Can you work these out from the model? Positions are in its coordinate system, mm. Face numbers are marked on the shaded views. A direction names the side the tool comes from. Coordinates: 2 decimals unless noted, no trailing zeros. Order: outer loops, then holes, each group sorted by start corner. A loop starts at its lowest first (then second) coordinate and runs counter-clockwise, first axis right, second up. Notation, with made-up numbers: (89, -26) -> (119, -26) arc R29 ccw to (119, 7) -> close; hole circle Ø8 at (-23, 13.5). An arc over 180 degrees is marked (long way). Answer in a Markdown table with one row per item. Add a question column.
1. Imagine slicing it at B-B on y = -21. Write out the boundary of the cut face in (x, z), plus the area to 3 significant figures.
2. Imagine slicing it at C-C on z = 4.75. Write out the boundary of the cut face in (x, y), plus the area to 3 significant figures.
3. Imagine slicing it at D-D on y = 5. Write out the boundary of the cut face in (x, z), plus the area to 3 significant figures.
4. On a 3-axis mill with a long thin cutter (end or side, diameter ignored), from which of +Z, -Z, +X, -X, +Y, -Y can I reach the whole of each face in a straight line? I mean the marked faces 1, 2, 3 and 4. Say none if no direction works.
5. Will these pins go through, and if not, where does the flat tip stop? pin 1 (6 mm diameter, centred on x = 17.5, y = -27, fed in from +Z); pin 2 (3 mm diameter, centred on x = -5.66, y = -5.66, fed in from +Z); pin 3 (1.8 mm diameter, centred on y = -2, z = 9, fed in from +X); pin 4 (3 mm diameter, centred on y = -24.5, z = 1.5, fed in from +X).
6. Imagine slicing it at A-A on x = 0. Write out the boundary of the cut face in (y, z), plus the area to 3 significant figures.
7. If I drill on line 1 along Y through (x, z) = (23.5, 22); line 2 along Z through (x, y) = (-8.5, -22); line 3 along Y through (x, z) = (-7, 4.75), over which ranges is the centre line in solid material (lowest first)? Write a range as [from, to].
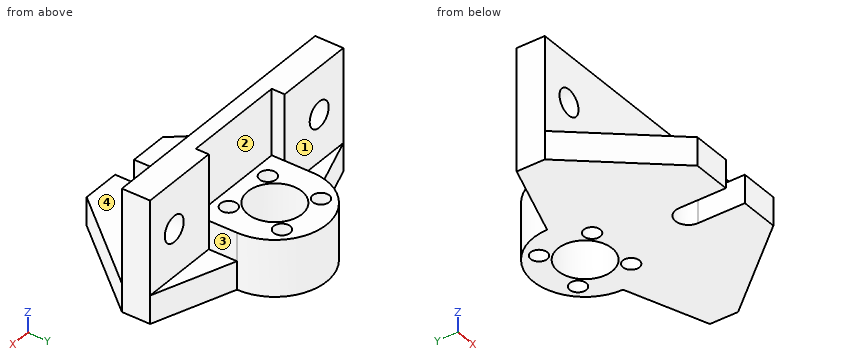
from build123d import *

# Parameters (mm, degrees)
SKETCH_R        = 5.75
SKETCH_R_2      = 1.75
PAD_DEPTH       = 26
SKETCH001_W     = 22
SKETCH001_H     = 6
PAD001_DEPTH    = 20
POCKET_DEPTH    = 6.001
PAD002_DEPTH    = 26
PAD002_FACE13_W = 20
PAD002_FACE13_H = 20
POCKET001_DEPTH = 144.217351
SKETCH004_R     = 2.75
POCKET002_DEPTH = 153.217351
POCKET003_DEPTH = 14
PAD003_DEPTH    = 6


with BuildPart() as part:
    # Sketch → Pad (new body)
    with BuildSketch(Plane.XY):
        with BuildLine():
            ThreePointArc((11, 0), (0, 11), (-11, 0))
            Line((-11, 0), (-11, -12))
            Line((11, -12), (-11, -12))
            Line((11, -12), (11, 0))
        make_face()
        Circle(SKETCH_R, mode=Mode.SUBTRACT)
        with Locations((-5.656854, 5.656854)):
            Circle(SKETCH_R_2, mode=Mode.SUBTRACT)
        with Locations((5.656854, -5.656854)):
            Circle(SKETCH_R_2, mode=Mode.SUBTRACT)
        with Locations((-5.656854, -5.656854)):
            Circle(SKETCH_R_2, mode=Mode.SUBTRACT)
        with Locations((5.656854, 5.656854)):
            Circle(SKETCH_R_2, mode=Mode.SUBTRACT)
    extrude(amount=PAD_DEPTH)

    # Sketch001 (on Face4 of Pad) → Pad001 (join)
    with BuildSketch(Plane.XZ.offset(12)):
        with Locations((0, 3)):
            Rectangle(SKETCH001_W, SKETCH001_H)
    extrude(amount=PAD001_DEPTH)

    # Sketch002 (on Face4 of Pad001) → Pocket (cut, through all)
    with BuildSketch(Plane.XY.offset(6)):
        with BuildLine():
            ThreePointArc((2.75, -22), (0, -19.25), (-2.75, -22))
            Line((-2.75, -22), (-2.75, -32))
            Line((-2.75, -32), (2.75, -32))
            Line((2.75, -22), (2.75, -32))
        make_face()
    extrude(amount=-POCKET_DEPTH, mode=Mode.SUBTRACT)

    # Sketch003 → Pad002 (join)
    with BuildSketch(Plane.XY):
        Polygon((11, -6), (28, -6), (28, -12), (11, -32), align=None)
    pad002 = extrude(amount=PAD002_DEPTH)

    # Pad002 Face13 → Pocket001 (cut, through all)
    with BuildSketch(Plane(origin=(11, -22, 16), x_dir=(0, 1, 0), z_dir=(-1, 0, 0))):
        Rectangle(PAD002_FACE13_W, PAD002_FACE13_H)
    pocket001 = extrude(amount=-POCKET001_DEPTH, mode=Mode.SUBTRACT)

    # Sketch004 (on Face6 of Pocket001) → Pocket002 (cut, through all)
    with BuildSketch(Plane(origin=(0, -6, 0), x_dir=(-1, 0, 0), z_dir=(0, 1, 0))):
        with Locations((-21, 16)):
            Circle(SKETCH004_R)
    pocket002 = extrude(amount=-POCKET002_DEPTH, mode=Mode.SUBTRACT)

    # Mirrored: Pad002, Pocket001, Pocket002 across Sketch003 V_Axis
    add(pad002.mirror(Plane(origin=(0, 0, 0), x_dir=(0, 0, 1), z_dir=(1, 0, 0))))
    add(pocket001.mirror(Plane(origin=(0, 0, 0), x_dir=(0, 0, 1), z_dir=(1, 0, 0))), mode=Mode.SUBTRACT)
    add(pocket002.mirror(Plane(origin=(0, 0, 0), x_dir=(0, 0, 1), z_dir=(1, 0, 0))), mode=Mode.SUBTRACT)

    # Sketch005 (on Face23 of Mirrored) → Pocket003 (cut)
    with BuildSketch(Plane.XY.offset(26)):
        with BuildLine():
            Line((-11, 0), (-11, -8.756854))
            Line((-11, -8.756854), (11, -8.756854))
            Line((11, -8.756854), (11, 0))
            ThreePointArc((11, 0), (0, 11), (-11, 0))
        make_face()
    extrude(amount=-POCKET003_DEPTH, mode=Mode.SUBTRACT)

    # Sketch006 (on Face2 of Pocket003) → Pad003 (join)
    with BuildSketch(Plane(origin=(0, 0, 0), x_dir=(1, 0, 0), z_dir=(0, 0, -1))):
        Polygon((-28, 6), (-11, 0), (-11, 6), align=None)
    pad003 = extrude(amount=-PAD003_DEPTH)

    # Mirrored001: Pad003 across Sketch006 V_Axis
    add(pad003.mirror(Plane(origin=(0, 0, 0), x_dir=(0, 0, -1), z_dir=(1, 0, 0))))


solid = part.part
Answers follow:
| question | item | result |
|---|---|---|
| 1 | outline | (-20.35, 0) -> (-2.56, 0) -> (-2.56, 6) -> (-20.35, 6) -> close; (2.56, 0) -> (20.35, 0) -> (20.35, 6) -> (2.56, 6) -> close |
| 1 | area | 213 mm² |
| 2 | outline | (-28, -12) -> (-11, -32) -> (-2.75, -32) -> (-2.75, -22) arc R2.75 cw to (2.75, -22) -> (2.75, -32) -> (11, -32) -> (28, -12) -> (28, -6) -> (11, 0) arc R11 ccw to (-11, 0) -> (-28, -6) -> close; hole circle Ø3.5 at (-5.66, -5.66); hole circle Ø3.5 at (-5.66, 5.66); hole circle Ø11.5 at (0, 0); hole circle Ø3.5 at (5.66, -5.66); hole circle Ø3.5 at (5.66, 5.66) |
| 2 | area | 1,330 mm² |
| 3 | outline | (-9.8, 0) -> (-7.28, 0) -> (-7.28, 12) -> (-9.8, 12) -> close; (-4.03, 0) -> (-2.84, 0) -> (-2.84, 12) -> (-4.03, 12) -> close; (2.84, 0) -> (4.03, 0) -> (4.03, 12) -> (2.84, 12) -> close; (7.28, 0) -> (9.8, 0) -> (9.8, 12) -> (7.28, 12) -> close |
| 3 | area | 89.1 mm² |
| 4 | face 1 | +Z, -X, +Y |
| 4 | face 2 | +Z, +Y |
| 4 | face 3 | +Z, +X, +Y |
| 4 | face 4 | +Z, +X, -X, -Y |
| 5 | pin 1 | stops at z = 6 |
| 5 | pin 2 | passes through |
| 5 | pin 3 | stops at x = 11 |
| 5 | pin 4 | stops at x = 18.65 |
| 6 | outline | (-19.25, 0) -> (-5.75, 0) -> (-5.75, 12) -> (-8.76, 12) -> (-8.76, 26) -> (-12, 26) -> (-12, 6) -> (-19.25, 6) -> close; (5.75, 0) -> (11, 0) -> (11, 12) -> (5.75, 12) -> close |
| 6 | area | 227 mm² |
| 7 | line 1 | y = [-12, -6] |
| 7 | line 2 | z = [0, 6] |
| 7 | line 3 | y = [-32, -6.78], [-4.54, 4.54], [6.78, 8.49] |
